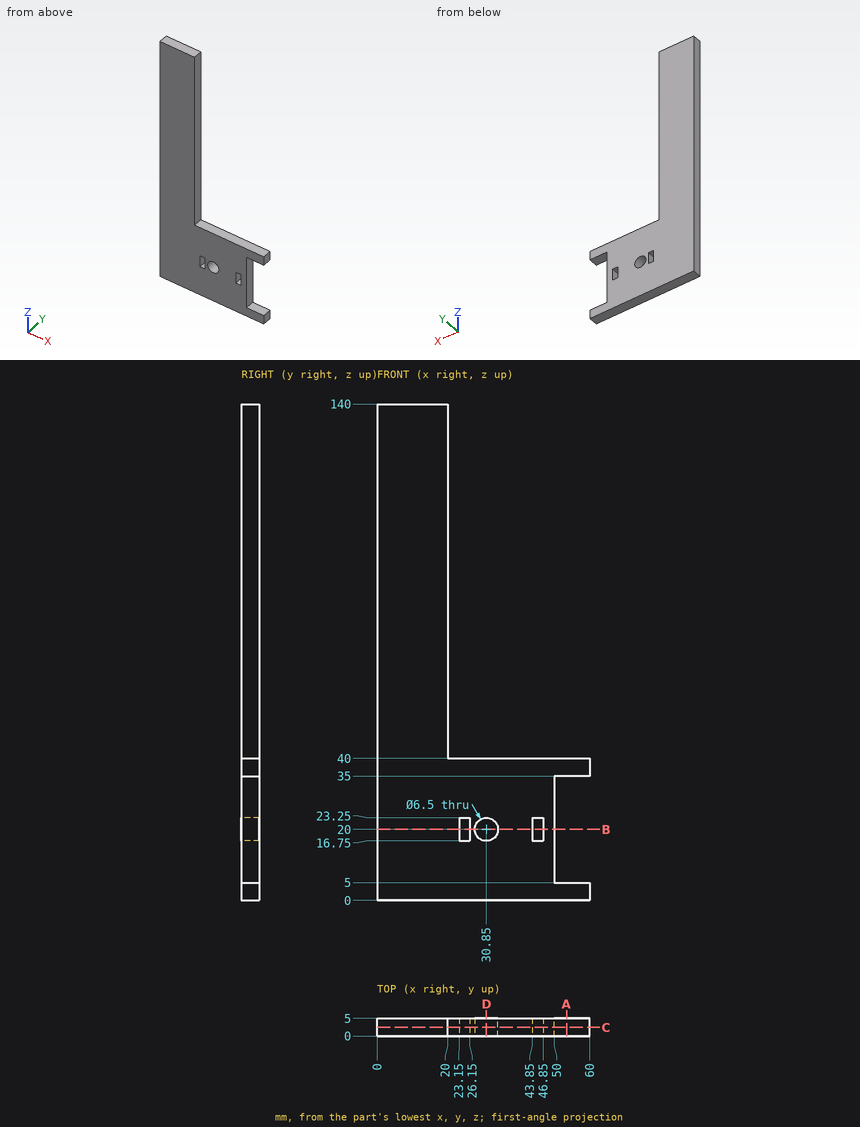
Input: dimensioned drawing with shaded views. Units: mm. Origin: part minimum x, y, z. Coordinates: 2 decimals unless noted, no trailing zeros. Write each loop counter-clockwise with the first axis right and the second up, starting at its lowest first coordinate (ties: lowest second). Pieces come first, ordered by that corner, then holes. Notation, with made-up numbers: M -17,55 L 10,55 A25 ccw 10,94 Z; hole C -27,-10.75 d9. An arc over 180 degrees is marked long. Answer as a JSON object with one key per item and string values. Group by question number.
(1) Section C-C on y = 2.45. Output: boundary loops of the cut face in (x, z).
(2) Section B-B on z = 20. Output: boundary loops of the cut face in (x, y), plus the area to 4 significant figures.
(3) Section A-A on x = 53.5. Output: boundary loops of the cut face in (y, z).
(4) Section D-D on x = 30.85. Output: boundary loops of the cut face in (y, z).
(5) Ray query, line 1 along X through (y, z) = (3.5, 20); line 2 along Z through (x, y) = (30.85, 1.95); line 3 along X through (y, z) = (4.75, 6.5). Return the intervals inside material, ascending. Write a range as [from, to].
(6) Contact query for a flat-ended pin moving along its axis: P1, Ø1, axis at x = 28, y = 1, coming from the +Z side. Output: stop coordinate, or through.
Result set:
{
 "1": {"outline": "M 0,0 L 60,0 L 60,5 L 50,5 L 50,35 L 60,35 L 60,40 L 20,40 L 20,140 L 0,140 Z; hole M 23.15,16.75 L 26.15,16.75 L 26.15,23.25 L 23.15,23.25 Z; hole C 30.85,20 d6.5; hole M 43.85,16.75 L 46.85,16.75 L 46.85,23.25 L 43.85,23.25 Z"},
 "2": {"outline": "M 0,0 L 23.15,0 L 23.15,5 L 0,5 Z; M 26.15,0 L 27.6,0 L 27.6,5 L 26.15,5 Z; M 34.1,0 L 43.85,0 L 43.85,5 L 34.1,5 Z; M 46.85,0 L 50,0 L 50,5 L 46.85,5 Z", "area": "187.5 mm2"},
 "3": {"outline": "M 0,0 L 5,0 L 5,5 L 0,5 Z; M 0,35 L 5,35 L 5,40 L 0,40 Z"},
 "4": {"outline": "M 0,0 L 5,0 L 5,16.75 L 0,16.75 Z; M 0,23.25 L 5,23.25 L 5,40 L 0,40 Z"},
 "5": {"line 1": "x = [0, 23.15], [26.15, 27.6], [34.1, 43.85], [46.85, 50]", "line 2": "z = [0, 16.75], [23.25, 40]", "line 3": "x = [0, 50]"},
 "6": {"P1": "stops at z = 40"}
}
